Model file for the job. Use its own axes, mm. Give positions to 0.01 mm unless a question says otherwise; leave off trailing zeros. Loops run counter-clockwise (first coordinate to the right, second up) from the corner with the lowest first, then second, coordinate; pieces in that order, holes last. Notation, with made-up numbers: M 20,-36 L 70,-36 A22 cw 70,-20 Z; hole C 88.25,44.25 d8. An arc over 180 degrees is marked long. Answer in a Markdown table with one row per item.
```python
from build123d import *

# Parameters (mm, degrees)
BASENUT_START         = -18
BASENUTSKE_R          = 8.75
BASENUT_DEPTH         = 18
SKETCH4_W             = 0.8
SKETCH4_H             = 12.629909152
IZIM1_W               = 62.269157962
IZIM1_H               = 48.757925573
KES_EKSTR_ZYON1_DEPTH = 6


# Read off the part's stored shape, not the designer's step: ThreadSchematic
with BuildPart() as part:
    # BaseNutSke → BaseNut (new body)
    with BuildSketch(Plane.XY.offset(BASENUT_START)):
        Polygon((17, 9.814954576), (17, -9.814954576), (0, -19.629909152), (-17, -9.814954576), (-17, 9.814954576), (0, 19.629909152), align=None)
        Circle(BASENUTSKE_R, mode=Mode.SUBTRACT)
    extrude(amount=BASENUT_DEPTH)

    # Sketch5 (on Front Plane) → EndChamfer (revolve, cut)
    with BuildSketch(Plane.XY):
        Polygon((17.9746, 10), (17.011814635, 8.625), (18.0254, 8.625), (18.0254, 10), align=None)
    revolve(axis=Axis((17.9746, 10, 0), (-0.5735764363510453, -0.8191520442889925, 0)), mode=Mode.SUBTRACT)

    # Sketch4 → Bearing-Face (revolve, cut)
    with BuildSketch(Plane(origin=(0, 0, 0), x_dir=(0, 0, -1), z_dir=(1, 0, 0)), mode=Mode.PRIVATE) as bearing_face_sk:
        with Locations((17.6, 23.314954576)):
            Rectangle(SKETCH4_W, SKETCH4_H)
        Polygon((0, 17), (-10, 17), (-10, 29.629909152), (1.518378757, 29.629909152), (1.518378757, 19.629909152), align=None)
    revolve(bearing_face_sk.sketch.rotate(Axis((0, 0, 0), (0, 0, -1)), 270), axis=Axis((0, 0, 0), (0, 0, -1)), mode=Mode.SUBTRACT)

    # ThreadSchematic outline → ThreadSchematic (revolve, cut)
    with BuildSketch(Plane.XZ):
        Polygon((8.75, 0), (8.75, -0.875259423), (10, 0), align=None)
        Polygon((10, -17.9746), (8.75, -17.099340577), (8.75, -18), (10, -18), align=None)
    revolve(axis=Axis((0, 0, 0), (0, 0, 1)), mode=Mode.SUBTRACT)

    # Çizim1 → Kes-Ekstrüzyon1 (cut)
    with BuildSketch(Plane(origin=(0, 0, -18), x_dir=(-1, 0, 0), z_dir=(0, 0, -1))):
        with Locations((0.923127679, 2.056057103)):
            Rectangle(IZIM1_W, IZIM1_H)
    extrude(amount=-KES_EKSTR_ZYON1_DEPTH, mode=Mode.SUBTRACT)


solid = part.part
```
(1) Mould opens along X. For faces 1 (the conical face through (-0.043, 17.627, -0.362)), 2 (the cylindrical face through (-6.944, -5.324, -6.516)), 3 (the flat face through (-7.3, -7.3, 0)), 4 (the conical face through (15.24, 8.85, -0.36)) say: pulls with the +X half, pulls with the -X half, needs draft (parallel to the pull), parting line crosses it, or undercut.
Established:
| item | result |
|---|---|
| face 1 | parting line crosses it |
| face 2 | undercut |
| face 3 | needs draft |
| face 4 | pulls with the +X half |
(2) Flat gauge pins, fed straight in: P1, Ø12, axis at x = 12.5, y = 9.5, coming from the +Z side; P2, Ø1.5, axis at x = 5.5, y = -5, coming from the -Z side; P3, Ø5, axis at x = -7, z = -2.5, coming from the -Y side; P4, Ø5, axis at x = -0.5, z = -7.5, coming from the +Y side. Where does each tip first touch, or does it go through?
Established:
| item | result |
|---|---|
| P1 | stops at z = 0 |
| P2 | passes through |
| P3 | stops at y = -17.03 |
| P4 | stops at y = 19.63 |
(3) Saw through at A-A, the plane z = -4.5. Give the cut face in (x, y), and give its area (3 significant figures).
Established:
| item | result |
|---|---|
| outline | M -17,-9.81 L 0,-19.63 L 17,-9.81 L 17,9.81 L 0,19.63 L -17,9.81 Z; hole C 0,0 d17.5 |
| area | 761 mm2 |
(4) Wall check: L1, parallel to X at y = 0, z = -9.25; L2, parallel to Y at x = 0, z = -4.75; L3, parallel to X at y = 5, z = -4. Give the ranges that are in metal, low to high.
Established:
| item | result |
|---|---|
| L1 | x = -17 to -8.75, 8.75 to 17 |
| L2 | y = -19.63 to -8.75, 8.75 to 19.63 |
| L3 | x = -17 to -7.18, 7.18 to 17 |
